Autodesk Inventor part; units mm, degrees
ref_plane "MidPlane" through (0, -71.2585, 3.048) normal (1, 0, 0) x (0, 0, -1)
ref_plane "YZ Plane" through (0, 0, 0) normal (1, 0, 0) x (0, 1, 0)
ref_plane "XZ Plane" through (0, 0, 0) normal (0, 1, 0) x (-1, 0, 0)
sketch "Base" plane through (0, 0, 0) normal (0, 0, 1) x (1, 0, 0)
  line L0 (-173.8499, -66.2658) -> (171.6188, -178.9186) construction
  line L1 (-9.525, -101.5493) -> (-9.525, 101.5493) construction
  line L2 (-9.525, 0) -> (-9.525, -119.85)
  line L3 (187.0398, -183.9472) -> (-9.525, -119.85)
  line L4 (187.0398, -183.9472) -> (187.0398, 0)
  line L5 (187.0398, 0) -> (-9.525, 0) construction
  line L6 (-9.525, 0) -> (-9.525, 119.85)
  line L7 (187.0398, 183.9472) -> (-9.525, 119.85)
  line L8 (187.0398, 183.9472) -> (187.0398, 0)
  point P0 (0, 0)
  point P1 (187.0398, -182.4643)
extrude "Plate1" add sketch "Base" along normal blind 3
sketch "MountHoles" plane through (0, 0, 0) normal (0, 0, -1) x (-1, 0, 0)
  line L0 (-179.0398, 172.9239) -> (1.525, 114.0441) construction
  circle A0 centre (-179.0398, 172.9239) radius 3
  circle A1 centre (1.525, 114.0441) radius 3
  line L1 (-226.3528, 0) -> (48.838, 0) construction
  circle A2 centre (-179.0398, -172.9239) radius 3
  circle A3 centre (1.525, -114.0441) radius 3
  line L2 (-187.0398, 183.9472) -> (9.525, 119.85)
  point P0 (0, 0)
  dimension "d2" = 6
  dimension "d3" = 6
  dimension "d45" = 8
extrude "MountHolesFeature" cut sketch "MountHoles" against normal blind 3
sketch "TorsoLiftMountHoles" plane through (0, 0, 3) normal (0, 0, 1) x (1, 0, 0)
  circle A0 centre (180.0398, -133.6037) radius 3
  circle A1 centre (164.0398, -133.6037) radius 3
  circle A2 centre (180.0398, 133.6037) radius 3
  circle A3 centre (164.0398, 133.6037) radius 3
  point P0 (0, 0)
extrude "TorsoLiftMountHolesFeature" cut sketch "TorsoLiftMountHoles" against normal blind 3
sketch "Continuation" plane through (0, 0, 0) normal (0, 0, -1) x (-1, 0, 0)
  line L0 (9.525, 119.85) -> (164.525, 69.3065)
  line L1 (-257.3528, 0) -> (234.838, 0) construction
  line L2 (9.525, -119.85) -> (164.525, -69.3065)
  line L3 (164.525, 69.3065) -> (164.525, -69.3065)
  line L4 (-187.0398, 183.9472) -> (9.525, 119.85)
  line L5 (9.525, 119.85) -> (9.525, -119.85)
  circle A0 centre (1.525, 114.0441) radius 3
  line L6 (1.525, 114.0441) -> (164.525, 60.8919) construction
  circle A1 centre (139.525, 69.0441) radius 3
  circle A2 centre (139.525, -69.0441) radius 3
  point P0 (0, 0)
  dimension "d46" = 155
  dimension "d47" = 25
sheet face with bend "ContinuationFeature" sketch "Continuation" thickness 3 toward (0, 0, 1) bend radius 3 contours L0 L3 L2 L5
bend "Bend2"
fillet "OutsideFilletsFeature" radius 8 4 edges at (187.0398, -183.9472, 1.5) (187.0398, 183.9472, 1.5) (-164.525, 69.3065, 1.5) (-164.525, -69.3065, 1.5)
ref_plane "MidPlane" through (0, -71.2585, 3.048) normal (1, 0, 0) x (0, 0, -1)
sketch "BottomMountHoles" plane through (0, 0, 0) normal (0, 0, -1) x (-1, 0, 0)
  circle A0 centre (18.4607, -50.75) radius 2.75
  circle A1 centre (18.4607, -8.25) radius 2.75
  circle A2 centre (18.4607, 8.25) radius 2.75
  circle A3 centre (18.4607, 50.75) radius 2.75
  ellipse E0 centre (103.3601, -25.3391) end of major axis (108.1225, -25.3596) minor radius 4.7625
  ellipse E1 centre (103.5793, 25.4605) end of major axis (108.3417, 25.4399) minor radius 4.7625
  spline S0 degree 3 poles (-22.2189, -83.25) (-22.5891, -83.25) (-22.9886, -83.178) (-23.6929, -82.9105) (-24.0824, -82.71) (-24.7238, -82.1045) (-24.9548, -81.7839) (-25.3958, -80.8943) (-25.4483, -80.428) (-25.4764, -79.9859) (-25.4838, -79.5156) (-25.1415, -78.5243) (-24.922, -78.15) (-24.3999, -77.5609) (-24.0923, -77.3244) (-23.5146, -77.014) (-23.2534, -76.9113) (-22.8383, -76.8067) (-22.5689, -76.75) (-22.2189, -76.75) knots 0 0 0 0 0.111053 0.111053 0.202489 0.202489 0.273701 0.273701 0.38581 0.38581 0.497395 0.497395 0.578796 0.578796 0.654724 0.654724 0.709985 0.709985 0.740525 0.740525 0.740525 0.740525 construction
  arc A4 (-22.2189, 83.25) -> (-22.2189, 76.75) centre (-22.2189, 80) ccw construction
  arc A5 (-133.7189, -83.25) -> (-133.7189, -76.75) centre (-133.7189, -80) ccw construction
  spline S1 degree 3 poles (-133.7189, 83.25) (-133.3487, 83.25) (-132.9492, 83.178) (-132.2449, 82.9105) (-131.8554, 82.71) (-131.2141, 82.1045) (-130.983, 81.7839) (-130.542, 80.8943) (-130.4896, 80.428) (-130.4615, 79.9859) (-130.4541, 79.5156) (-130.7963, 78.5243) (-131.0158, 78.15) (-131.538, 77.5609) (-131.8456, 77.3244) (-132.4232, 77.014) (-132.6845, 76.9113) (-133.0996, 76.8067) (-133.3689, 76.75) (-133.7189, 76.75) knots 0 0 0 0 0.111053 0.111053 0.202489 0.202489 0.273701 0.273701 0.38581 0.38581 0.497395 0.497395 0.578796 0.578796 0.654725 0.654725 0.709986 0.709986 0.740527 0.740527 0.740527 0.740527 construction
  line L0 (167.4427, 0) -> (-246.1203, 0) construction
  point P0 (0, 0)
extrude "Cut8" cut sketch "BottomMountHoles" against normal blind 3 contours E0 | E1
delete faces "Delete1" heal yes whole lump no faces at (-139.4042, 72.0417, 2) (-4.5153, 113.8027, 2) (179.1606, 175.9215, 2) (179.1606, -169.9264, 2) (-4.5153, -114.2855, 2) (-139.4042, -66.0465, 2)
sketch "Sketch15" plane through (187.0398, -172.9239, 3) normal (0, 0, 1) x (1, 0, 0)
  line L0 (-346.045, 244.0304) -> (-10.4802, 353.4537)
  line L1 (-346.045, 244.0304) -> (-0.3836, 348.2954)
  line L2 (-423.7471, 172.9239) -> (72.8866, 172.9239) construction
  line L3 (0, 345.8479) -> (0, 0)
  arc A0 (0, 345.8479) -> (-10.4802, 353.4537) centre (-8, 345.8479) ccw
  arc A1 (-346.045, 244.0304) -> (-351.5648, 236.4246) centre (-343.5648, 236.4246) ccw
  line L4 (-351.5648, 109.4233) -> (-351.5648, 236.4246)
  line L5 (-346.045, 101.8175) -> (-0.3836, -2.4475)
  arc A2 (-10.4802, -7.6058) -> (0, 0) centre (-8, 0) ccw
  line L6 (-10.4802, -7.6058) -> (-346.045, 101.8175)
  arc A3 (-351.5648, 109.4233) -> (-346.045, 101.8175) centre (-343.5648, 109.4233) ccw
  point P0 (-187.0398, 172.9239)
  dimension "d84" = 178.725
extrude "AdjustToProductionFeature" cut sketch "Sketch15" against normal blind 3 contours L0 A0 L1 | L5 A2 L6
delete faces "Delete2" heal yes whole lump no faces at (187.0208, 173.4763, 1) (187.0208, -173.4763, 2)
fillet "Fillet5" radius 6 2 edges at (187.0398, 175.4872, 1.5) (187.0398, -175.4872, 1.5)
sketch "ContactorMount" plane through (-164.525, -63.5006, 0) normal (0, 0, -1) x (-1, 0, 0)
  circle A0 centre (-109.3281, 40.5006) radius 2.25
  circle A1 centre (-109.3281, 86.5006) radius 2.25
  point P0 (-164.525, 63.5006)
extrude "Cut12" cut sketch "ContactorMount" against normal blind 3
sketch "Sketch19" plane through (-164.525, -63.5006, 0) normal (0, 0, -1) x (-1, 0, 0)
  line L0 (-332.5315, 63.5006) -> (-247.3998, 15.1574)
  line L1 (-247.3998, 15.1574) -> (-247.3998, 111.8439)
  line L2 (-247.3998, 111.8439) -> (-332.5315, 63.5006)
  line L3 (-332.5315, 82.9372) -> (-247.3998, 131.2805)
  line L4 (-247.3998, 131.2805) -> (-332.5315, 177.8709)
  line L5 (-332.5315, 177.8709) -> (-332.5315, 82.9372)
  line L6 (-351.5648, -103.9097) -> (-351.5648, 230.9109)
  line L7 (-351.5648, 63.5006) -> (0, 63.5006) construction
  line L8 (0, 0) -> (0, 127.0012)
  line L9 (-332.5315, 63.5006) -> (-332.5315, 82.9372) construction
  line L10 (-247.3998, 111.8439) -> (-247.3998, 131.2805) construction
  line L11 (-332.5315, 44.064) -> (-247.3998, -4.2792)
  line L12 (-247.3998, -4.2792) -> (-332.5315, -50.8696)
  line L13 (-332.5315, -50.8696) -> (-332.5315, 44.064)
  point P0 (-164.525, 63.5006)
  point P1 (-247.3998, 63.5006)
extrude "Cut13" cut sketch "Sketch19" against normal blind 3
fillet "Fillet8" radius 6 9 edges at (168.0065, -19.4366, 1.5) (168.0065, -114.3703, 1.5) (82.8748, -67.7798, 1.5) (82.8748, -48.3432, 1.5) (168.0065, 0, 1.5) (82.8748, 48.3432, 1.5) (168.0065, 19.4366, 1.5) (82.8748, 67.7798, 1.5) (168.0065, 114.3703, 1.5)
equation "\"d7\" = Thickness"
equation "\"d43\" = Thickness"
equation "\"d82\" = Thickness"
equation "\"d85\" = Thickness"
equation "\"d0\" = Thickness"
equation "\"d48\" = BendRadius"
equation "\"d49\" = BendReliefWidth"
equation "\"d51\" = MinimumRemnant"
equation "\"d50\" = BendReliefDepth"
equation "\"d52\" = TransitionRadius"
equation "\"BendRadius\" = Thickness"
equation "\"BendReliefWidth\" = Thickness"
equation "\"BendReliefDepth\" = 0.5 * Thickness"
equation "\"CornerReliefSize\" = 4 * Thickness"
equation "\"MinimumRemnant\" = 2 * Thickness"
equation "\"TransitionRadius\" = BendRadius"
equation "\"JacobiRadiusSize\" = BendRadius"
equation "\"GapSize\" = Thickness"
CAD build for the part. Positions are in the model's coordinates, mm. A direction names the side the tool comes from. Coordinates: 2 decimals unless noted, no trailing zeros. Order: outer loops, then holes, each group sorted by start corner. A loop starts at its lowest first (then second) coordinate and runs counter-clockwise, first axis right, second up.
Item 1: Band-saw the part on B-B on y = -9.5. List the corners of the cut face in (x, z) (3 decimals), plus the area to 3 significant figures.
Check sheet entries:
outline: (-164.525, 0) - (82.875, 0) - (82.875, 3) - (-164.525, 3) - close; (151.277, 0) - (187.04, 0) - (187.04, 3) - (151.277, 3) - close
area: 849 mm2
Item 2: Band-saw the part on C-C on z = 2.3. Give the number of separate pieces and of enclosed holes in the cut face, plus the area to 3 significant figures.
Check sheet entries:
separate pieces: 1
enclosed holes: 11
area: 73,800 mm2
Item 3: Two-plate mould, pull along Y, no slides. Class faces 1 (the face through (125.3, -91, 1.5)), 2 (the face through (7.783, 121.416, 1.521)), 3 (the face through (125.797, -23.969, 1.479)), 4 (the face through (14, 2, 0)): +Y half, -Y half, draft (parallel to the pull), parting line (faces both ways), or undercut.
Check sheet entries:
face 1: undercut
face 2: +Y half
face 3: undercut
face 4: draft
Item 4: 3-axis set-ups, long thin cutter, end or side, ignore diameter. For faces 5 (the face through (14, 2, 3)), 6 (the face through (126.11, -43.23, 1.48)): which of +Z, -Z, +X, -X, +Y, -Y reach the whole face in a straight line?
Check sheet entries:
face 5: +Z, +X, -X, +Y, -Y
face 6: +Z, -Z
Item 5: Band-saw the part on D-D on y = 121. List the corners of the cut face in (x, z), plus the area to 3 significant figures.
Check sheet entries:
outline: (6.4, 0) - (187.04, 0) - (187.04, 3) - (6.4, 3) - close
area: 542 mm2
Item 6: Drill centre lines: L1, parallel to X at y = 22, z = 1.85 (3 decimals); L2, parallel to Y at x = 131.5, z = 2.4; L3, parallel to Y at x = -105, z = 1.8. Where is each one in solid material? Low to high.
Check sheet entries:
L1: x = -164.525 to -106.851, -100.307 to -57.212, -53.181 to 82.875, 129.265 to 187.04
L2: y = -158.73 to -94.39, -40.17 to -20.73, 20.73 to 40.17, 94.39 to 158.73
L3: y = -87.4 to -29.81, -20.87 to 20.91, 30.01 to 87.4
Item 7: Band-saw the part on A-A on y = 79.5. List the corners of the cut face in (x, z), plus the area to 3 significant figures.
Check sheet entries:
outline: (-131.18, 0) - (104.29, 0) - (104.29, 3) - (-131.18, 3) - close; (168.01, 0) - (187.04, 0) - (187.04, 3) - (168.01, 3) - close
area: 764 mm2
